from build123d import *

# Parameters (mm, degrees)
F0_W     = 215.9
F0_H     = 19.05
F1_DEPTH = 7.9375
F2_SIZE2 = 19.04999
F2_SIZE  = 19.04999
F3_SIZE2 = 19.04999
F3_SIZE  = 19.04999


# Not quite as in the source:
# - a fillet or chamfer is up to 0.001 mm smaller than in the source, because OpenCascade refuses the exact size


with BuildPart() as f1:
    # F0 (on Right) → F1 (new body, symmetric)
    with BuildSketch(Plane.YZ):
        Rectangle(F0_W, F0_H)
    extrude(amount=F1_DEPTH, both=True)

    # F2 (size 19.05 and 19.05 in the source; OpenCascade refuses exactly that, so slightly less here)
    f2_edges = [f1.edges().sort_by_distance(p)[0] for p in [
        (0, -107.95, 9.525),
    ]]
    chamfer(f2_edges, length=F2_SIZE, length2=F2_SIZE2)

    # F3 (size 19.05 and 19.05 in the source; OpenCascade refuses exactly that, so slightly less here)
    f3_edges = [f1.edges().sort_by_distance(p)[0] for p in [
        (0, 107.95, 9.525),
    ]]
    chamfer(f3_edges, length=F3_SIZE, length2=F3_SIZE2)


solid = f1.part
Geometry: final body of the model. Coordinates: model frame, mm. Coordinates: 2 decimals unless noted, no trailing zeros. Write each loop counter-clockwise with the first axis right and the second up, starting at its lowest first coordinate (ties: lowest second). Pieces come first, ordered by that corner, then holes. Notation, with made-up numbers: (-5.5, -20) - (27.5, -20) arc R30 cw to (27.5, 19) - close; hole circle Ø1 at (-29, 28). An arc over 180 degrees is marked (long way). Return JSON: item names as keys, results as strings.
Item 1: Section query B-B (z = -5.5). Output: boundary loops of the cut face in (x, y), and give its area (3 significant figures).
Completed:
{"outline": "(-7.94, -103.93) - (7.94, -103.93) - (7.94, 103.93) - (-7.94, 103.93) - close", "area": "3,300 mm2"}
Item 2: Line query: L1, parallel to Y at x = 0.25, z = 8.25; L2, parallel to Y at x = 2.25, z = 8. Output: solid intervals per line, ascending.
Completed:
{"L1": "y = -90.18 to 90.18", "L2": "y = -90.43 to 90.43"}
Item 3: Section query C-C (z = 6.75). Output: boundary loops of the cut face in (x, y).
Completed:
{"outline": "(-7.94, -91.68) - (7.94, -91.68) - (7.94, 91.68) - (-7.94, 91.68) - close"}
Item 4: Pin query (flat end, axial travel): pin 1 Ø2 at (x, z) = (-6, -0.5) entering from -Y (3 decimals); pin 2 Ø1 at (x, z) = (6, 3.5) entering from -Y (3 decimals); pin 3 Ø5 at (x, z) = (6, 5.5) entering from +Y (3 decimals). Return the tip coordinate at first contact, or that it passes through.
Completed:
{"pin 1": "stops at y = -99.925", "pin 2": "stops at y = -95.425", "pin 3": "stops at y = 95.425"}
